The listing builds one solid part. Answer for the finished solid, in the listing's coordinates (mm). A direction names the side the tool comes from. Round coordinates to 2 decimals unless told otherwise and drop trailing zeros. Order: outer loops, then holes, each group sorted by start corner. A loop starts at its lowest first (then second) coordinate and runs counter-clockwise, first axis right, second up. Notation, with made-up numbers: (27.25, 0.5) - (78.25, 0.5) arc R28 ccw to (78.25, 32.5) - close; hole circle Ø4 at (-3, 60.25). An arc over 180 degrees is marked (long way). One line per item, written item: value. Start each with the question number.
1. Section C-C, the plane x = -11.5 is taken. Give the vertices of the cut face in (y, z), then the cut area to 3 significant figures.
2. Flat-ended cylindrical pins translate along their axes: P1, Ø4, axis at y = 79.5, z = 32.5, coming from the -X side; P2, Ø5, axis at x = -15, y = 77, coming from the -Z side; P3, Ø4, axis at y = 78.5, z = 28, coming from the +X side. Find the tip coordinate at first contact, or state that the pin passes through.
3. Section A-A, the plane y = 78 is taken. Give the vertices of the cut face in (x, z).
4. Section B-B, the plane z = 16 is taken. Give the vertices of the cut face in (x, y), then the cut area to 3 significant figures.
5. Section D-D, the plane x = -26 is taken. Give the vertices of the cut face in (y, z), then the cut area to 3 significant figures.
6. Straight lines are drawn through the part: line 1 (X direction, y = 84.5, z = -1); line 2 (X direction, y = 80.25, z = 7); line 3 (Z direction, x = -1.5, y = 78.25). For each, find the intervals that lie inside material, in ascending order.
7. A tool of negligible diameter and unlimited length cuts with its end or side. For faces 4 (the flat face through (0, 79, 33)), 5 (the flat face through (-25, 79, 34)), 6 (the flat face through (-23, 79, 0)), from which of +Z, -Z, +X, -X, +Y, -Y can it reach the whole face along a straight path? Write none if from no direction.
8. For a pull along X with two mould halves and no side action, classify faces 1 (the cylindrical face through (-25.76, 79.06, 14.49)), 2 (the cylindrical face through (0.802, 79.06, 13.441)), 3 (the flat face through (-2, 79, 0)) as released by +X, released by -X, zero draft, split by the parting line, or undercut.
from build123d import *

# Parameters (mm, degrees)
SKETCH1_W           = 3.85
SKETCH1_H           = 12.714938244
BOSS_EXTRUDE1_DEPTH = 50
BOSS_EXTRUDE2_DEPTH = 12.714938244
SKETCH4_W           = 19.052451889
SKETCH4_H           = 12.714938244
BOSS_EXTRUDE3_DEPTH = 3
FILLET1_R           = 10
SKETCH5_W           = 19.999198202
SKETCH5_H           = 12.714938244
BOSS_EXTRUDE4_DEPTH = 3
FILLET2_R           = 10


with BuildPart() as part:
    # Sketch1 → Boss-Extrude1 (new body)
    with BuildSketch(Plane.XY):
        with Locations((-23.075, 79.148527214)):
            Rectangle(SKETCH1_W, SKETCH1_H)
    extrude(amount=BOSS_EXTRUDE1_DEPTH)

    # Sketch3 → Boss-Extrude2 (add)
    with BuildSketch(Plane(origin=(0, 85.505996336, 0), x_dir=(1, 0, 0), z_dir=(0, 1, 0))):
        Polygon((-21.15, -45.165463377), (-3.42398491, -45.165463377), (-3.42398491, 0), (0, 0), (0, -50), (-21.15, -50), align=None)
    extrude(amount=-BOSS_EXTRUDE2_DEPTH)

    # Sketch4 → Boss-Extrude3 (add)
    with BuildSketch(Plane(origin=(0, 0, 0), x_dir=(0, 0, -1), z_dir=(1, 0, 0))):
        with Locations((-0.697437539, 79.148527214)):
            Rectangle(SKETCH4_W, SKETCH4_H)
    extrude(amount=BOSS_EXTRUDE3_DEPTH)

    # Fillet1
    # the kernel refuses this fillet: 10 mm, written as the material it adds along each edge
    with BuildSketch(Plane(origin=(0, 72.791058092, 10.223663483), x_dir=(0, 0, 1), z_dir=(0, 1, 0))) as fillet1_piece_1:
        with BuildLine():
            CenterArc((7.141428429, 10), FILLET1_R, 224.427004001, 45.572995999)
            Line((0, 3), (-0.142828569, 2.86))
            ThreePointArc((-0.142828569, 2.86), (-0.2, 1.5), (-0.2, 0))
            Line((-0.2, 0), (0, -0.2))
            Line((0, -0.2), (7.141428429, -0.2))
            Line((7.141428429, -0.2), (7.141428429, 0))
        make_face()
    extrude(amount=12.714938244)

    # Sketch5 → Boss-Extrude4 (add)
    with BuildSketch(Plane.ZY.offset(25)):
        with Locations((1.170810695, 79.148527214)):
            Rectangle(SKETCH5_W, SKETCH5_H)
    extrude(amount=BOSS_EXTRUDE4_DEPTH)

    # Fillet2
    # the kernel refuses this fillet: 10 mm, written as the material it adds along each edge
    with BuildSketch(Plane(origin=(-25, 72.791058092, 11.170409796), x_dir=(0, 0, 1), z_dir=(0, 1, 0))) as fillet2_piece_1:
        with BuildLine():
            CenterArc((7.141428429, -10), FILLET2_R, 90, 45.572995999)
            Line((0, -3), (-0.142828569, -2.86))
            ThreePointArc((-0.142828569, -2.86), (-0.2, -1.5), (-0.2, 0))
            Line((-0.2, 0), (0, 0.2))
            Line((0, 0.2), (7.141428429, 0.2))
            Line((7.141428429, 0.2), (7.141428429, 0))
        make_face()
    extrude(amount=12.714938244)


solid = part.part
Answer list:
1. outline: (72.79, 45.17) - (85.51, 45.17) - (85.51, 50) - (72.79, 50) - close
1. area: 61.5 mm²
2. P1: stops at x = -25
2. P2: stops at z = 45.17
2. P3: stops at x = 0
3. outline: (-28, -8.83) - (-25, -8.83) - (-25, 0) - (-21.15, 0) - (-21.15, 45.17) - (-3.42, 45.17) - (-3.42, 0) - (0, 0) - (0, -8.83) - (3, -8.83) - (3, 10.22) arc R10 cw to (0, 17.37) - (0, 50) - (-25, 50) - (-25, 18.31) arc R10 cw to (-28, 11.17) - close
4. outline: (-25.27, 72.79) - (-21.15, 72.79) - (-21.15, 85.51) - (-25.27, 85.51) - close; (-3.42, 72.79) - (0.09, 72.79) - (0.09, 85.51) - (-3.42, 85.51) - close
4. area: 97.1 mm²
5. outline: (72.79, -8.83) - (85.51, -8.83) - (85.51, 13.95) - (72.79, 13.95) - close
5. area: 290 mm²
6. line 1: x = -28 to -25, 0 to 3
6. line 2: x = -28 to -21.15, -3.42 to 3
6. line 3: z = 0 to 50
7. face 4: +Z, +X, +Y, -Y
7. face 5: +Z, -X, +Y, -Y
7. face 6: -Z, +Y, -Y
8. face 1: released by -X
8. face 2: released by +X
8. face 3: undercut
